Autodesk Inventor part; units mm, degrees
ref_plane "YZ Plane" through (0, 0, 0) normal (1, 0, 0) x (0, 1, 0)
ref_plane "XZ Plane" through (0, 0, 0) normal (0, 1, 0) x (-1, 0, 0)
ref_plane "XY Plane" through (0, 0, 0) normal (0, 0, 1) x (1, 0, 0)
sketch "Sketch1" plane through (0, 0, 0) normal (0, 0, 1) x (1, 0, 0)
  circle A0 centre (0, 0) radius 11
  line L0 (-26, -15) -> (26, -15)
  line L1 (26, -15) -> (26, 15)
  line L2 (-26, 15) -> (-26, -15)
  circle A1 centre (0, 0) radius 16 construction
  circle A2 centre (11.3137, 11.3137) radius 2
  circle A3 centre (-11.3137, -11.3137) radius 2
  circle A4 centre (11.3137, -11.3137) radius 2
  circle A5 centre (-11.3137, 11.3137) radius 2
  circle A6 centre (-16, 0) radius 2
  circle A7 centre (16, 0) radius 2
  line L3 (-11.3137, 11.3137) -> (0, 0) construction
  line L4 (0, 0) -> (-16, 0) construction
  line L5 (-26, 15) -> (26, 15)
  point P0 (0, -15)
  dimension "d0" = 22
  dimension "d2" = 52
  dimension "d3" = 32
  dimension "d4" = 4
  dimension "d5" = 45
  dimension "d6" = 15
  dimension "d16" = 30
extrude "Extrusion1" add sketch "Sketch1" along normal blind 36
sketch "Sketch3" plane through (-26, 15, 0) normal (0, 1, 0) x (1, 0, 0)
  circle A0 centre (8.5, -6) radius 2.5
  circle A1 centre (43.5, -6) radius 2.5
  circle A2 centre (43.5, -30) radius 2.5
  circle A3 centre (8.5, -30) radius 2.5
  line L0 (8.5, -6) -> (43.5, -6) construction
  line L1 (43.5, -6) -> (43.5, -30) construction
  line L2 (43.5, -30) -> (8.5, -30) construction
  line L3 (8.5, -30) -> (8.5, -6) construction
  line L4 (52, 0) -> (0, 0) construction
  line L5 (52, 0) -> (52, -36) construction
  point P0 (26, 0)
  point P1 (26, -6)
  point P2 (26, 0)
  point P3 (43.5, -18)
  point P4 (52, -18)
  dimension "d17" = 5
  dimension "d18" = 35
  dimension "d19" = 24
extrude "Extrusion3" cut sketch "Sketch3" against normal blind 10
properties part number "DSG16H"
Model file for the job. Use its own axes, mm. A direction names the side the tool comes from. Round coordinates to 2 decimals unless told otherwise and drop trailing zeros. Loops run counter-clockwise (first coordinate to the right, second up) from the corner with the lowest first, then second, coordinate; pieces in that order, holes last. Notation, with made-up numbers: (58.5, 55) - (80.5, 55) arc R13 cw to (80.5, 78) - close; hole circle Ø4 at (79, 55.25). An arc over 180 degrees is marked (long way). Write each question's results on one line, items separated by ' | '.
(1) Wall check: L1, parallel to Z at x = -17.5, y = 8.25; L2, parallel to X at y = -10, z = 34.5; L3, parallel to Y at x = 12, z = 19. Give the ranges that are in metal, low to high.
Answer below:
L1: z = 0 to 3.5, 8.5 to 27.5, 32.5 to 36 | L2: x = -26 to -12.82, -9.81 to -4.58, 4.58 to 9.81, 12.82 to 26 | L3: y = -15 to -13.19, -9.44 to 9.44, 13.19 to 15
(2) Saw through at B-B, the plane x = 16. List the corners of the cut face in (y, z), then the cut area to 3 significant figures.
Answer below:
outline: (-15, 0) - (-2, 0) - (-2, 36) - (-15, 36) - close; (2, 0) - (15, 0) - (15, 4) - (5, 4) - (5, 8) - (15, 8) - (15, 28) - (5, 28) - (5, 32) - (15, 32) - (15, 36) - (2, 36) - close | area: 856 mm^2
(3) 3-axis set-ups, long thin cutter, end or side, ignore diameter. For faces 5 (the cylindrical face through (16, 10, 28)), 6 (the flat face through (-26, 0, 18)): which of +Z, -Z, +X, -X, +Y, -Y reach the whole face in a straight line?
Answer below:
face 5: +Y | face 6: +Z, -Z, -X, +Y, -Y
(4) Pin check, flat tips, straight feed: pin 1 (5 mm diameter, centred on x = -18, y = -6.5, fed in from -Z); pin 2 (2.5 mm diameter, centred on x = 17.5, z = 30, fed in from +Y). Stop position of each tip, or through.
Answer below:
pin 1: stops at z = 0 | pin 2: stops at y = 5
(5) Saw through at D-D, the plane z = 22. List the corners of the cut face in (x, y), then the cut area to 3 significant figures.
Answer below:
outline: (-26, -15) - (26, -15) - (26, 15) - (-26, 15) - close; hole circle Ø4 at (-16, 0); hole circle Ø4 at (-11.31, -11.31); hole circle Ø4 at (-11.31, 11.31); hole circle Ø22 at (0, 0); hole circle Ø4 at (11.31, -11.31); hole circle Ø4 at (11.31, 11.31); hole circle Ø4 at (16, 0) | area: 1,100 mm^2
(6) Saw through at C-C, the plane y = 0. List the corners of the cut face in (x, z), then the cut area to 3 significant figures.
Answer below:
outline: (-26, 0) - (-18, 0) - (-18, 36) - (-26, 36) - close; (-14, 0) - (-11, 0) - (-11, 36) - (-14, 36) - close; (11, 0) - (14, 0) - (14, 36) - (11, 36) - close; (18, 0) - (26, 0) - (26, 36) - (18, 36) - close | area: 792 mm^2
(7) Saw through at A-A, the plane y = 10.25. List the corners of the cut face in (x, z).
Answer below:
outline: (-26, 0) - (-13.01, 0) - (-13.01, 36) - (-26, 36) - close; (-9.62, 0) - (-3.99, 0) - (-3.99, 36) - (-9.62, 36) - close; (3.99, 0) - (9.62, 0) - (9.62, 36) - (3.99, 36) - close; (13.01, 0) - (26, 0) - (26, 36) - (13.01, 36) - close; hole circle Ø5 at (-17.5, 6); hole circle Ø5 at (-17.5, 30); hole circle Ø5 at (17.5, 6); hole circle Ø5 at (17.5, 30)
(8) Mould opens along Z. For faces 1 (the cylindrical face through (15, 10, 6)), 2 (the flat face through (-6, 10, 36)), 3 (the flat face through (17, 5, 6)), 4 (the cylindrical face through (-9.466, -10.548, 17.748)) say: released by +Z, released by -Z, zero draft, split by the parting line, or undercut.
Answer below:
face 1: undercut | face 2: released by +Z | face 3: undercut | face 4: zero draft
